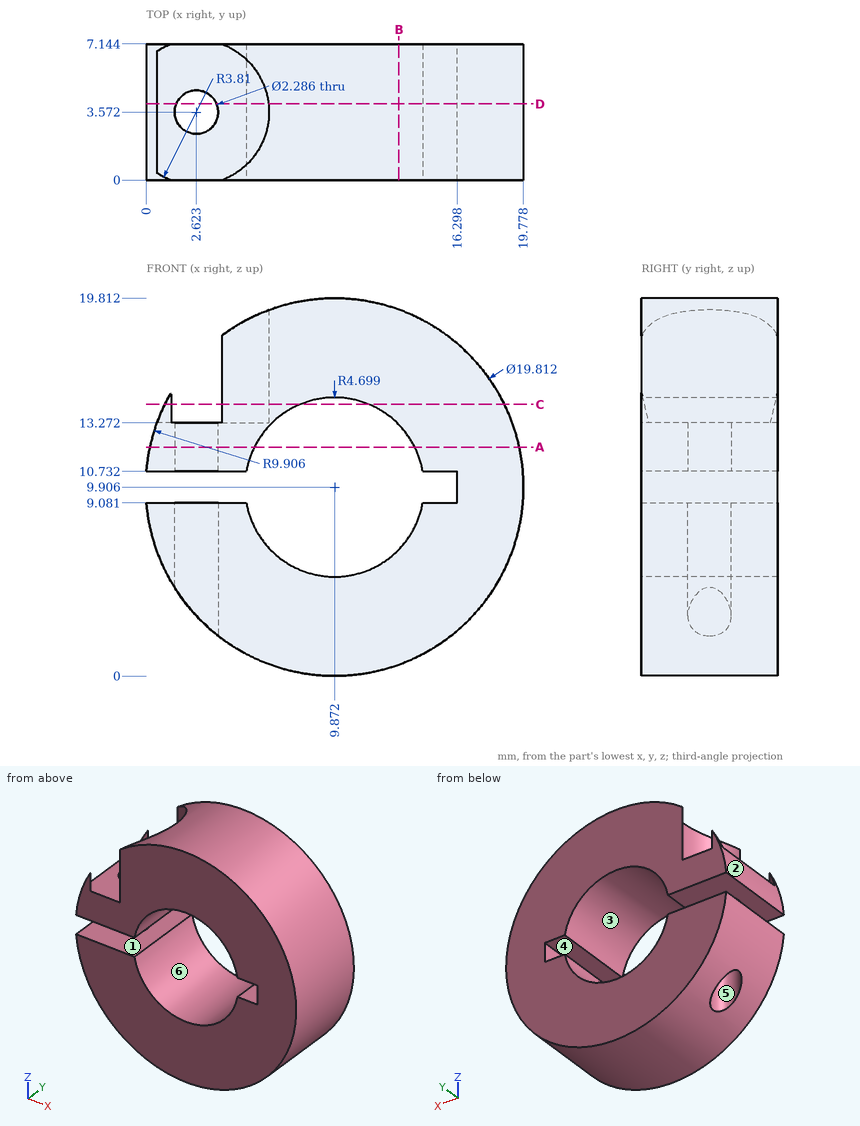
Could you check a few things on this drawing? It's one solid part, dimensions in mm from its lowest x, y, z. A direction names the side the tool comes from. Round coordinates to 2 decimals unless told otherwise and drop trailing zeros. Write each loop counter-clockwise with the first axis right and the second up, starting at its lowest first coordinate (ties: lowest second). Pieces come first, ordered by that corner, then holes. Notation, with made-up numbers: (15.25, 16.25) -> (23.25, 16.25) arc R29 ccw to (23.25, 52.25) -> close; hole circle Ø4 at (-23, 39.25). An arc over 180 degrees is marked (long way). Use a Markdown table: item, result.
1. Please list where these lines run through material, in increasing order: probe 1 along X at (y, z) = (2.75, 12.75) (1 decimal); probe 2 along X at (y, z) = (1.25, 13.5) (1 decimal); probe 3 along Z at (x, y) = (8.5, 4.75) (1 decimal).
Answer key:
| item | result |
|---|---|
| probe 1 | x = 0.4 to 1.8, 3.4 to 6.1, 13.6 to 19.4 |
| probe 2 | x = 5.6 to 6.8, 12.9 to 19.1 |
| probe 3 | z = 0.1 to 5.4, 14.4 to 19.7 |
2. If we section it at B-B (x = 13.25): List the corners of the cut face in (y, z) for me.
Answer key:
| item | result |
|---|---|
| outline | (0, 0.59) -> (7.14, 0.59) -> (7.14, 6.64) -> (0, 6.64) -> close; (0, 13.17) -> (7.14, 13.17) -> (7.14, 19.22) -> (0, 19.22) -> close |
3. If we section it at D-D (y = 4): List the corners of the cut face in (x, z) for me (1 decimal), then the cut area to 3 significant figures.
Answer key:
| item | result |
|---|---|
| outline | (0, 9.1) arc R9.9 ccw to (1.6, 4.5) -> (1.6, 9.1) -> close; (0, 10.7) -> (1.6, 10.7) -> (1.6, 13.3) -> (0.6, 13.3) arc R9.9 ccw to start; (3.7, 2.2) arc R9.9 ccw (long way) to (6.4, 19.2) -> (6.4, 13.3) -> (3.7, 13.3) -> (3.7, 10.7) -> (5.2, 10.7) arc R4.7 cw to (14.5, 10.7) -> (16.3, 10.7) -> (16.3, 9.1) -> (14.5, 9.1) arc R4.7 cw to (5.2, 9.1) -> (3.7, 9.1) -> close |
| area | 187 mm^2 |
4. We'd pull the mould along X, two halves only. Please class the marked faces 1, 2 and 3: +X half, -X half, draft (parallel to the pull), parting line (faces both ways), or undercut.
Answer key:
| item | result |
|---|---|
| face 1 | draft |
| face 2 | -X half |
| face 3 | undercut |
5. If we section it at A-A (z = 12): List the corners of the cut face in (x, y) for me (1 decimal).
Answer key:
| item | result |
|---|---|
| outline | (0.2, 0) -> (5.7, 0) -> (5.7, 7.1) -> (0.2, 7.1) -> close; (14.1, 0) -> (19.6, 0) -> (19.6, 7.1) -> (14.1, 7.1) -> close; hole circle Ø2.3 at (2.6, 3.6) |
6. For pin 1 Ø4 at (y, z) = (2, 7) entering from +X; pin 2 Ø4 at (x, y) = (2.5, 3) entering from +Z; pin 3 Ø0.5 at (x, y) = (15.5, 4) entering from +Z (1 decimal), each with a flat end and sliding along its axis, tell me the tip position at first contact or that it passes through.
Answer key:
| item | result |
|---|---|
| pin 1 | stops at x = 19.74 |
| pin 2 | stops at z = 13.27 |
| pin 3 | stops at z = 18.2 |
7. Which directions (+Z, -Z, +X, -X, +Y, -Y) give clear straight access to the entire face, cutting with the end or side of a thin tool? Please do the marked faces 4, 5 and 6.
Answer key:
| item | result |
|---|---|
| face 4 | -X, +Y, -Y |
| face 5 | +Z, -Z |
| face 6 | +Y, -Y |
8. If we section it at C-C (z = 14.25): State how many separate pieces and enclosed holes the cut face has.
Answer key:
| item | result |
|---|---|
| separate pieces | 4 |
| enclosed holes | 0 |
